```python
from build123d import *

# Parameters (mm, degrees)
BOSS_EXTRUDE1_DEPTH = 5.588
SKETCH3_R           = 1.3462
CUT_EXTRUDE2_DEPTH  = 5.588
CAVITY1_START       = 83.185
CAVITY1_DEPTH       = 31.115
CAVITY1_START_2     = -114.3
CAVITY1_2_DEPTH     = 31.115
CAVITY1_START_3     = 114.3
CAVITY1_3_DEPTH     = 4.318
CAVITY1_START_4     = -118.618
CAVITY1_4_DEPTH     = 4.318
CAVITY1_START_5     = 118.618
CAVITY1_5_DEPTH     = 4.8514


# Read off the part's stored shape, not the designer's step: Cavity1
with BuildPart() as part:
    # Sketch1 → Boss-Extrude1 (new body)
    with BuildSketch(Plane.XY):
        with BuildLine():
            Line((65.305122421, -132.260512242), (132.260512242, -65.305122421))
            ThreePointArc((132.260512242, -65.305122421), (137.766540126, -57.064769361), (139.7, -47.344610179))
            Line((139.7, -47.344610179), (139.7, 78.378975516))
            ThreePointArc((139.7, 78.378975516), (137.766540126, 88.099134698), (132.260512242, 96.339487758))
            Line((132.260512242, 96.339487758), (96.339487758, 132.260512242))
            ThreePointArc((96.339487758, 132.260512242), (88.099134698, 137.766540126), (78.378975516, 139.7))
            Line((78.378975516, 139.7), (-78.378975516, 139.7))
            ThreePointArc((-78.378975516, 139.7), (-88.099134698, 137.766540126), (-96.339487758, 132.260512242))
            Line((-96.339487758, 132.260512242), (-132.260512242, 96.339487758))
            ThreePointArc((-132.260512242, 96.339487758), (-137.766540126, 88.099134698), (-139.7, 78.378975516))
            Line((-139.7, 78.378975516), (-139.7, -47.344610179))
            ThreePointArc((-139.7, -47.344610179), (-137.766540126, -57.064769361), (-132.260512242, -65.305122421))
            Line((-132.260512242, -65.305122421), (-65.305122421, -132.260512242))
            ThreePointArc((-65.305122421, -132.260512242), (-57.064769361, -137.766540126), (-47.344610179, -139.7))
            Line((-47.344610179, -139.7), (47.344610179, -139.7))
            ThreePointArc((47.344610179, -139.7), (57.064769361, -137.766540126), (65.305122421, -132.260512242))
        make_face()
    extrude(amount=BOSS_EXTRUDE1_DEPTH)

    # Sketch3 → Cut-Extrude2 (cut)
    with BuildSketch(Plane(origin=(0, 0, 0), x_dir=(-1, 0, 0), z_dir=(0, 0, -1))):
        with Locations((-32.4104, 19.658336728)):
            Circle(SKETCH3_R)
        with Locations((35.687, 19.745836517)):
            Circle(SKETCH3_R)
        with Locations((28.0416, -55.144663272)):
            Circle(SKETCH3_R)
        with Locations((-25.2984, -54.636663272)):
            Circle(SKETCH3_R)
    extrude(amount=-CUT_EXTRUDE2_DEPTH, mode=Mode.SUBTRACT)

    # Cavity1 outline → Cavity1 (cut)
    with BuildSketch(Plane.YZ.offset(CAVITY1_START)):
        with BuildLine():
            ThreePointArc((-30.161375078, 5.588), (-31.865780452, 2.863110305), (-33.326130038, 0))
            Line((-33.326130038, 0), (33.689150844, 0))
            ThreePointArc((33.689150844, 0), (32.228801258, 2.863110305), (30.524395884, 5.588))
            Line((30.524395884, 5.588), (-30.161375078, 5.588))
        make_face()
    extrude(amount=CAVITY1_DEPTH, mode=Mode.SUBTRACT)

    # Cavity1 2 outline → Cavity1 2 (cut)
    with BuildSketch(Plane.YZ.offset(CAVITY1_START_2)):
        with BuildLine():
            Line((-33.347208643, 0), (33.347208643, 0))
            ThreePointArc((33.347208643, 0), (31.84705315, 2.865329857), (30.101301452, 5.588))
            Line((30.101301452, 5.588), (-30.101301452, 5.588))
            ThreePointArc((-30.101301452, 5.588), (-31.84705315, 2.865329857), (-33.347208643, 0))
        make_face()
    extrude(amount=CAVITY1_2_DEPTH, mode=Mode.SUBTRACT)

    # Cavity1 3 outline → Cavity1 3 (cut)
    with BuildSketch(Plane.YZ.offset(CAVITY1_START_3)):
        with BuildLine():
            ThreePointArc((-11.660862641, 5.588), (-15.245647335, 3.098030401), (-18.320194056, 0))
            Line((-18.320194056, 0), (18.683214863, 0))
            ThreePointArc((18.683214863, 0), (15.608668142, 3.098030401), (12.023883447, 5.588))
            Line((12.023883447, 5.588), (-11.660862641, 5.588))
        make_face()
    extrude(amount=CAVITY1_3_DEPTH, mode=Mode.SUBTRACT)

    # Cavity1 4 outline → Cavity1 4 (cut)
    with BuildSketch(Plane.YZ.offset(CAVITY1_START_4)):
        with BuildLine():
            ThreePointArc((-11.208900442, 5.588), (-14.972228516, 3.12349524), (-18.209542122, 0))
            Line((-18.209542122, 0), (18.209542122, 0))
            ThreePointArc((18.209542122, 0), (14.972228516, 3.12349524), (11.208900442, 5.588))
            Line((11.208900442, 5.588), (-11.208900442, 5.588))
        make_face()
    extrude(amount=CAVITY1_4_DEPTH, mode=Mode.SUBTRACT)

    # Cavity1 5 outline → Cavity1 5 (cut)
    with BuildSketch(Plane.YZ.offset(CAVITY1_START_5)):
        with BuildLine():
            ThreePointArc((3.456513242, 0), (0.181510403, 0.346877829), (-3.093492436, 0))
            Line((-3.093492436, 0), (3.456513242, 0))
        make_face()
    extrude(amount=CAVITY1_5_DEPTH, mode=Mode.SUBTRACT)


solid = part.part
```
For this review, take the finished solid that the model builds, in its own axes (mm). Give positions to 0.01 mm unless a question says otherwise; leave off trailing zeros. Write each loop counter-clockwise with the first axis right and the second up, starting at its lowest first coordinate (ties: lowest second). Pieces come first, ordered by that corner, then holes.
Item 1: Take a section at D-D (x = -68.5). Give the boundary of the cut face in (y, z).
Item 2: Wall thickness on probe 1 along X at (y, z) = (8, 0.55) (3 decimals); probe 2 along X at (y, z) = (-30, 2.05) (3 decimals); probe 3 along Y at (x, z) = (104.5, 3.15): over which ranges is each line inside the solid? List them lowest first.
Item 3: Take a section at B-B (y = 123). Give the boundary of the cut face in (x, z).
Item 4: Take a section at A-A (y = -23). Give the boundary of the cut face in (x, z) (3 decimals), and give its area (3 significant figures).
Item 5: Insertion check: P1, Ø2.5, axis at x = 32.41, y = 19.66, coming from the -Z side; P2, Ø1.5, axis at y = 92, z = 4.5, coming from the +X side; P3, Ø3, axis at x = -97.5, z = 3.5, coming from the +Y side. Each pin has a flat end and moves straight along its axis. Give the tip position at first contact, or say it passes through.
Item 6: Take a section at C-C (z = 1.3). Give the number of separate pieces and of enclosed holes in the cut face, and give its area (3 significant figures).
Established:
1. outline: (-129.07, 0) - (139.7, 0) - (139.7, 5.59) - (-129.07, 5.59) - close
2. probe 1: x = -139.7 to -118.618, -83.185 to 83.185, 118.618 to 139.7
2. probe 2: x = -139.7 to -114.3, -83.185 to 83.185, 114.3 to 139.7
2. probe 3: y = -93.07 to -31.7, 32.06 to 124.1
3. outline: (-105.6, 0) - (105.6, 0) - (105.6, 5.59) - (-105.6, 5.59) - close
4. outline: (-139.7, 0) - (-114.3, 0) - (-114.3, 5.588) - (-139.7, 5.588) - close; (-83.185, 0) - (83.185, 0) - (83.185, 5.588) - (-83.185, 5.588) - close; (114.3, 0) - (139.7, 0) - (139.7, 5.588) - (114.3, 5.588) - close
4. area: 1,210 mm2
5. P1: passes through
5. P2: stops at x = 136.2
5. P3: stops at y = 132.59
6. separate pieces: 1
6. enclosed holes: 6
6. area: 64,300 mm2
